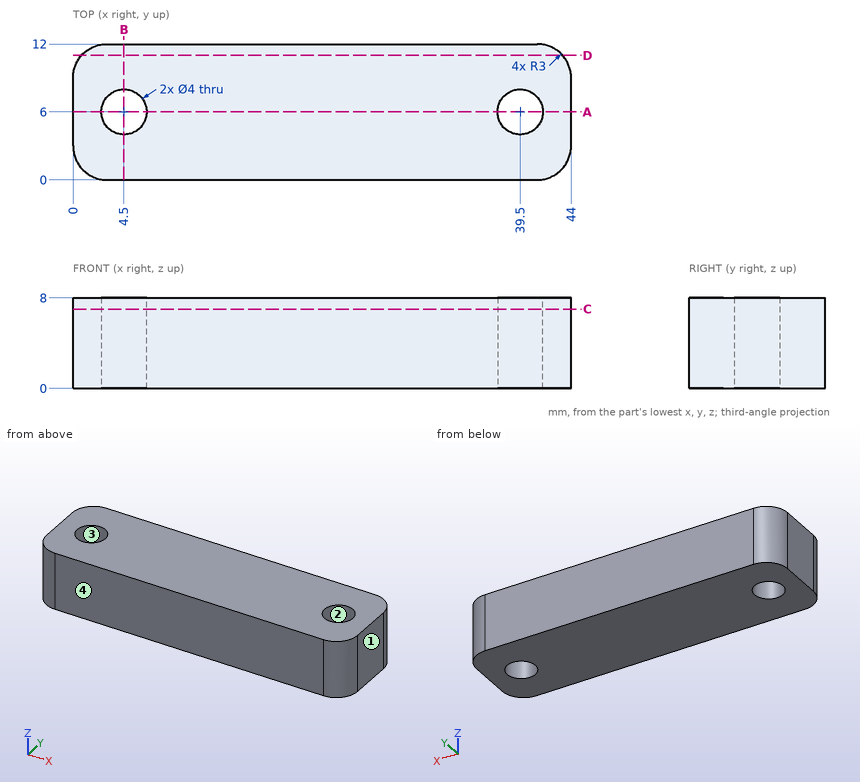
Part print with two shaded views. Sizes in mm from the minimum x, y, z corner. Round coordinates to 2 decimals unless told otherwise and drop trailing zeros. Order: outer loops, then holes, each group sorted by start corner. A loop starts at its lowest first (then second) coordinate and runs counter-clockwise, first axis right, second up. Notation, with made-up numbers: (9.5, -11) - (37.5, -11) arc R11 ccw to (37.5, 6) - close; hole circle Ø2 at (44, -6). An arc over 180 degrees is marked (long way). Return JSON: item names as keys, results as strings.
(1) Cut at D-D (y = 11). Give the cut face in (x, z).
Answer key:
{"outline": "(0.76, 0) - (43.24, 0) - (43.24, 8) - (0.76, 8) - close"}
(2) Cut at B-B (x = 4.5). Give the cut face in (y, z), then the cut area to 3 significant figures.
Answer key:
{"outline": "(0, 0) - (4, 0) - (4, 8) - (0, 8) - close; (8, 0) - (12, 0) - (12, 8) - (8, 8) - close", "area": "64.0 mm^2"}
(3) Pin check, flat tip, straight feed: pin 1 Ø6.5 at (x, y) = (39.5, 6) entering from -Z. Stop position of the tip, or through.
Answer key:
{"pin 1": "stops at z = 0"}
(4) Wall check: probe 1 along X at (y, z) = (6, 4.75); probe 2 along Y at (x, z) = (4.5, 4); probe 3 along X at (y, z) = (5.5, 2). Give the ranges that are in metal, low to high. Write a range as from..to.
Answer key:
{"probe 1": "x = 0..2.5, 6.5..37.5, 41.5..44", "probe 2": "y = 0..4, 8..12", "probe 3": "x = 0..2.56, 6.44..37.56, 41.44..44"}
(5) Cut at A-A (y = 6). Give the cut face in (x, z), then the cut area to 3 significant figures.
Answer key:
{"outline": "(0, 0) - (2.5, 0) - (2.5, 8) - (0, 8) - close; (6.5, 0) - (37.5, 0) - (37.5, 8) - (6.5, 8) - close; (41.5, 0) - (44, 0) - (44, 8) - (41.5, 8) - close", "area": "288 mm^2"}
(6) Cut at C-C (z = 7). Give the cut face in (x, y), then the cut area to 3 significant figures.
Answer key:
{"outline": "(0, 3) arc R3 ccw to (3, 0) - (41, 0) arc R3 ccw to (44, 3) - (44, 9) arc R3 ccw to (41, 12) - (3, 12) arc R3 ccw to (0, 9) - close; hole circle Ø4 at (4.5, 6); hole circle Ø4 at (39.5, 6)", "area": "495 mm^2"}
(7) Pull direction X, two halves, no side cores. Call the marked faces 1, 2, 3 and 4: +X half, -X half, draft (parallel to the pull), parting line (faces both ways), or undercut.
Answer key:
{"face 1": "+X half", "face 2": "undercut", "face 3": "undercut", "face 4": "draft"}
